The model under review builds one solid part; all positions refer to its coordinate system, in mm. Face numbers are marked on the shaded views. A direction names the side the tool comes from. Round coordinates to 2 decimals unless told otherwise and drop trailing zeros. Order: outer loops, then holes, each group sorted by start corner. A loop starts at its lowest first (then second) coordinate and runs counter-clockwise, first axis right, second up. Notation, with made-up numbers: (78.25, 24) -> (116.25, 24) arc R18 ccw to (116.25, 39) -> close; hole circle Ø4 at (-5, -35.5). An arc over 180 degrees is marked (long way). Use a Markdown table: item, result. Add a question column.
```python
from build123d import *

# Parameters (mm, degrees)
SKETCH1_R          = 3.3274
EXTRUDE3_DEPTH     = 2.1082
SKETCH4_W          = 4.2418
SKETCH4_H          = 1.7526
LPATTERN2_COUNT    = 5
LPATTERN2_PITCH    = 0.79375
SKETCH15_W         = 6.6548
SKETCH15_H         = 0.83185
CUT_EXTRUDE5_DEPTH = 1.0541


with BuildPart() as part:
    # Sketch1 → Extrude3 (new body)
    with BuildSketch(Plane.XY):
        Circle(SKETCH1_R)
    extrude(amount=EXTRUDE3_DEPTH)

    # Sketch11 → Cut-Revolve3 (revolve, cut)
    with BuildSketch(Plane(origin=(0, 0, 0), x_dir=(0, 0, -1), z_dir=(1, 0, 0))):
        Polygon((0, 1.494769699), (-2.1082, 3.3274), (0, 3.3274), align=None)
    revolve(axis=Axis((0, 0, -0.441444004), (0, 0, 1)), mode=Mode.SUBTRACT)

    # Sketch4 → Revolve1 (revolve)
    with BuildSketch(Plane(origin=(0, 0, 0), x_dir=(0, 0, -1), z_dir=(1, 0, 0))):
        with Locations((2.1209, 0.8763)):
            Rectangle(SKETCH4_W, SKETCH4_H)
    revolve(axis=Axis((0, 0, -4.2418), (0, 0, -1)))

    # Sketch5 → Cut-Revolve1 (revolve, cut)
    with BuildSketch(Plane(origin=(0, 0, 0), x_dir=(0, 0, -1), z_dir=(1, 0, 0))):
        Polygon((0.096768654, 1.774513192), (0.433577192, 1.410275607), (0.6271145, 1.454101991), (0.774149232, 1.927905533), align=None)
    cut_revolve1 = revolve(axis=Axis((0, -0.193538035, 0), (0, 0.220857364, -0.975306119)), mode=Mode.SUBTRACT)

    # Sketch13 → Cut-Revolve4 (revolve, cut)
    with BuildSketch(Plane(origin=(0, 0, 0), x_dir=(0, 0, -1), z_dir=(1, 0, 0))):
        Polygon((4.2418, 1.410275607), (3.507682971, 1.7526), (4.2418, 1.7526), align=None)
    revolve(axis=Axis((0, 0, 0), (0, 0, -1)), mode=Mode.SUBTRACT)

    # Sketch16 → Cut-Revolve5 (revolve, cut)
    with BuildSketch(Plane(origin=(0, 0, 0), x_dir=(0, 0, -1), z_dir=(1, 0, 0))):
        Polygon((0, 1.494769699), (0.708382929, 1.7526), (0, 1.7526), align=None)
    revolve(axis=Axis((0, 0, 0), (0, 0, -1)), mode=Mode.SUBTRACT)

    # LPattern2: Cut-Revolve1 ×5
    with Locations(*[(0, 0, -i * LPATTERN2_PITCH) for i in range(1, LPATTERN2_COUNT)]):
        add(cut_revolve1, mode=Mode.SUBTRACT)

    # Sketch15 → Cut-Extrude5 (cut)
    with BuildSketch(Plane.XY.offset(2.1082)):
        Rectangle(SKETCH15_W, SKETCH15_H)
    extrude(amount=-CUT_EXTRUDE5_DEPTH, mode=Mode.SUBTRACT)


solid = part.part
```
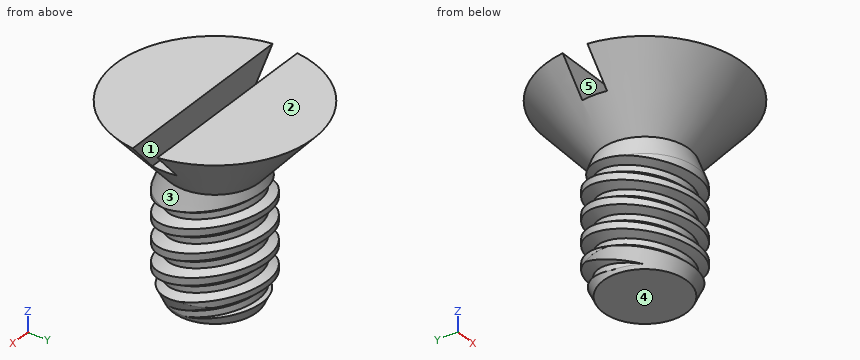
Q1. Wall thickness on line 1 (Y direction, x = -2, z = 1.25); line 2 (Z direction, x = -1, y = 0); line 3 (Y direction, x = 0.25, z = 0.5): over which ranges is each line inside the solid? List them lowest first. Write a range as [from, to].
Q2. Add section B-B (z = 0.5). Write out the cut boundary in (x, y).
Q3. Mouldability with a two-part tool opening along Z and no side actions: class the marked faces 3, 4 and 5 as pulls with the +Z half, pulls with the -Z half, needs draft (parallel to the pull), parting line crosses it, or undercut.
Q4. Add section A-A (z = 1.25). Write out the cut boundary in (x, y), then the cut area to 3 significant figures.
Q5. Machinability: for the marked faces 1 and 2, which of the approach directions +Z, -Z, +X, -X, +Y, -Y give a long, thin tool a straight path to every point of the face, cutting with its end or side? Answer none if there is none.
Q6. Insertion check: pin 1 (0.8 mm diameter, centred on x = -0.5, z = 1.5, fed in from -Y); pin 2 (0.7 mm diameter, centred on x = 1, y = 0, fed in from +Z); pin 3 (1 mm diameter, centred on x = -1.5, z = -3, fed in from -Y). Each pin has a flat end and moves straight along its axis. Give the tip position at first contact, or say it passes through.
Report:
| question | item | result |
|---|---|---|
| 1 | line 1 | y = [-1.63, -0.42], [0.42, 1.63] |
| 1 | line 2 | z = [-4.24, 1.05] |
| 1 | line 3 | y = [-1.91, 1.91] |
| 2 | outline | circle Ø3.86 at (0, 0) |
| 3 | face 3 | undercut |
| 3 | face 4 | pulls with the -Z half |
| 3 | face 5 | needs draft |
| 4 | outline | (-2.55, -0.42) arc R2.58 ccw to (2.55, -0.42) -> close; (-2.55, 0.42) -> (2.55, 0.42) arc R2.58 ccw to start |
| 4 | area | 16.7 mm² |
| 5 | face 1 | +Z, +X, -X |
| 5 | face 2 | +Z, +X, -X, +Y, -Y |
| 6 | pin 1 | stops at y = -3.11 |
| 6 | pin 2 | stops at z = 1.05 |
| 6 | pin 3 | stops at y = -1.43 |
